```python
from build123d import *

# Parameters (mm, degrees)
CROQUIS1_R              = 27.1
CROQUIS1_R_2            = 2.5
CROQUIS1_W              = 3
CROQUIS1_H              = 36
SALIENTE_EXTRUIR1_DEPTH = 2
CROQUIS2_R              = 28.1
CROQUIS2_R_2            = 27.1
SALIENTE_EXTRUIR2_DEPTH = 5


with BuildPart() as part:
    # Croquis1 → Saliente-Extruir1 (new body)
    with BuildSketch(Plane.XY):
        with BuildLine():
            Line((-56.5, 20), (-29.632119398, 20))
            ThreePointArc((-29.632119398, 20), (0, 35.75), (29.632119398, 20))
            Line((29.632119398, 20), (56.5, 20))
            Line((56.5, 20), (56.5, -20))
            Line((56.5, -20), (29.632119398, -20))
            ThreePointArc((29.632119398, -20), (0, -35.75), (-29.632119398, -20))
            Line((-29.632119398, -20), (-56.5, -20))
            Line((-56.5, -20), (-56.5, 20))
        make_face()
        Circle(CROQUIS1_R, mode=Mode.SUBTRACT)
        with Locations((31.5, 0)):
            Circle(CROQUIS1_R_2, mode=Mode.SUBTRACT)
        with Locations((22.273863607, -22.273863607)):
            Circle(CROQUIS1_R_2, mode=Mode.SUBTRACT)
        with Locations((0, -31.5)):
            Circle(CROQUIS1_R_2, mode=Mode.SUBTRACT)
        with Locations((-22.273863607, -22.273863607)):
            Circle(CROQUIS1_R_2, mode=Mode.SUBTRACT)
        with Locations((-31.5, 0)):
            Circle(CROQUIS1_R_2, mode=Mode.SUBTRACT)
        with Locations((-22.273863607, 22.273863607)):
            Circle(CROQUIS1_R_2, mode=Mode.SUBTRACT)
        with Locations((0, 31.5)):
            Circle(CROQUIS1_R_2, mode=Mode.SUBTRACT)
        with Locations((22.273863607, 22.273863607)):
            Circle(CROQUIS1_R_2, mode=Mode.SUBTRACT)
        with Locations((-48, 0)):
            Rectangle(CROQUIS1_W, CROQUIS1_H, mode=Mode.SUBTRACT)
        with Locations((-53, 0)):
            Rectangle(CROQUIS1_W, CROQUIS1_H, mode=Mode.SUBTRACT)
        with Locations((-43, 0)):
            Rectangle(CROQUIS1_W, CROQUIS1_H, mode=Mode.SUBTRACT)
        with Locations((-38, 0)):
            Rectangle(CROQUIS1_W, CROQUIS1_H, mode=Mode.SUBTRACT)
        with Locations((38, 0)):
            Rectangle(CROQUIS1_W, CROQUIS1_H, mode=Mode.SUBTRACT)
        with Locations((43, 0)):
            Rectangle(CROQUIS1_W, CROQUIS1_H, mode=Mode.SUBTRACT)
        with Locations((48, 0)):
            Rectangle(CROQUIS1_W, CROQUIS1_H, mode=Mode.SUBTRACT)
        with Locations((53, 0)):
            Rectangle(CROQUIS1_W, CROQUIS1_H, mode=Mode.SUBTRACT)
    extrude(amount=SALIENTE_EXTRUIR1_DEPTH)

    # Croquis2 → Saliente-Extruir2 (add)
    with BuildSketch(Plane.XY.offset(2)):
        Circle(CROQUIS2_R)
        Circle(CROQUIS2_R_2, mode=Mode.SUBTRACT)
    extrude(amount=SALIENTE_EXTRUIR2_DEPTH)


solid = part.part
```
Source: CAD feature listing. Evaluate the final solid. Frame: model axes, mm. A direction names the side the tool comes from. Give positions to 0.01 mm unless a question says otherwise; leave off trailing zeros. Order: outer loops, then holes, each group sorted by start corner. A loop starts at its lowest first (then second) coordinate and runs counter-clockwise, first axis right, second up. Notation, with made-up numbers: (-18, 73.25) -> (18, 73.25) arc R24 cw to (18, 90.25) -> close; hole circle Ø2 at (-7, 7.5). An arc over 180 degrees is marked (long way). Use a Markdown table: item, result.
Q1. Access query for faces 1 (the face through (-24.258, 20.753, 0.986)), 2 (the face through (-6.092, -27.432, 4.465)). Directions: +Z, -Z, +X, -X, +Y, -Y. A direction counts if a zero-diameter tool reaches every point of the face in a straight line with its end or side. Return the directions, or none.
A:
| item | result |
|---|---|
| face 1 | +Z, -Z |
| face 2 | +Z |
Q2. Section C-C (y = -31.5). Return the cut outline in (x, z).
A:
| item | result |
|---|---|
| outline | (-16.91, 0) -> (-2.5, 0) -> (-2.5, 2) -> (-16.91, 2) -> close; (2.5, 0) -> (16.91, 0) -> (16.91, 2) -> (2.5, 2) -> close |
Q3. Section B-B (x = 31.5). Return the cut outline in (y, z), and give its area (3 significant figures).
A:
| item | result |
|---|---|
| outline | (-20, 0) -> (-2.5, 0) -> (-2.5, 2) -> (-20, 2) -> close; (2.5, 0) -> (20, 0) -> (20, 2) -> (2.5, 2) -> close |
| area | 70.0 mm^2 |
Q4. Material intervals for line 1 (X direction, y = 1, z = 6.5); line 2 (Y direction, x = -31.5, z = 0.9); line 3 (X direction, y = 23.5, z = 4.75), sorted ascending. Write a range as [from, to].
A:
| item | result |
|---|---|
| line 1 | [-28.08, -27.08], [27.08, 28.08] |
| line 2 | [-20, -2.5], [2.5, 20] |
| line 3 | [-15.41, -13.5], [13.5, 15.41] |
Q5. Section D-D (z = 3.25). Return the cut outline in (x, y).
A:
| item | result |
|---|---|
| outline | circle Ø56.2 at (0, 0); hole circle Ø54.2 at (0, 0) |
Q6. First-contact query: P1, Ø2, axis at y = -23.5, z = 1, coming from the +X side; P2, Ø1.6, axis at x = 53.5, z = 1.5, coming from the -Y side; P3, Ø1, axis at y = 7.5, z = 3, coming from the +X side; P4, Ø3, axis at x = 31.5, y = 0, coming from the +Z side. Flat tips, straight axial feed; report the tip coordinate or a pass-through.
A:
| item | result |
|---|---|
| P1 | x = 27.78 |
| P2 | y = -20 |
| P3 | x = 27.21 |
| P4 | through |
Q7. Pull-direction query (X, two-part tool) for faces 3 (the face through (25.4, -10.4, 0)), 4 (the face through (-0.489, 35.747, 0.986)), 5 (the face through (0, -29, 1)); classes: +X half, -X half, draft (parallel to the pull), parting line (faces both ways), or undercut.
A:
| item | result |
|---|---|
| face 3 | draft |
| face 4 | parting line |
| face 5 | undercut |
Q8. Section A-A (x = 0). Return the cut outline in (y, z), and give its area (3 significant figures).
A:
| item | result |
|---|---|
| outline | (-35.75, 0) -> (-34, 0) -> (-34, 2) -> (-35.75, 2) -> close; (-29, 0) -> (-27.1, 0) -> (-27.1, 7) -> (-28.1, 7) -> (-28.1, 2) -> (-29, 2) -> close; (27.1, 0) -> (29, 0) -> (29, 2) -> (28.1, 2) -> (28.1, 7) -> (27.1, 7) -> close; (34, 0) -> (35.75, 0) -> (35.75, 2) -> (34, 2) -> close |
| area | 24.6 mm^2 |
